from build123d import *

# Parameters (mm, degrees)
SKETCH1_W           = 40
SKETCH1_H           = 40
SKETCH1_R           = 0.9
BOSS_EXTRUDE1_DEPTH = 6
SKETCH11_W          = 40
SKETCH11_H          = 40
SKETCH11_R          = 5
BOSS_EXTRUDE6_DEPTH = 7
SKETCH13_R          = 1.5
SKETCH13_R_2        = 1.395390764
CUT_EXTRUDE5_DEPTH  = 27
SKETCH13_3_R        = 3
SKETCH13_3_R_2      = 1.5
CUT_EXTRUDE6_DEPTH  = 3


with BuildPart() as part:
    # Sketch1 → Boss-Extrude1 (new body)
    with BuildSketch(Plane(origin=(0, 0, 0), x_dir=(0, 1, 0), z_dir=(0, 0, 1))):
        Rectangle(SKETCH1_W, SKETCH1_H)
        with Locations(Location((10.5, 0, 0), (0, 0, 270))):
            Circle(SKETCH1_R, mode=Mode.SUBTRACT)
        with Locations(Location((-10.5, 12.5, 0), (0, 0, 270))):
            Circle(SKETCH1_R, mode=Mode.SUBTRACT)
        with Locations(Location((-10.5, 0, 0), (0, 0, 270))):
            Circle(SKETCH1_R, mode=Mode.SUBTRACT)
        with Locations(Location((10.5, 12.5, 0), (0, 0, 270))):
            Circle(SKETCH1_R, mode=Mode.SUBTRACT)
        Polygon((-5, -13), (-8, -13), (-8, -5), (-5, -5), (-5, 5), (5, 5), (5, -5), (5, -13), align=None, mode=Mode.SUBTRACT)
    extrude(amount=BOSS_EXTRUDE1_DEPTH)

    # Sketch11 → Boss-Extrude6 (add)
    with BuildSketch(Plane.XY.offset(6)):
        Rectangle(SKETCH11_W, SKETCH11_H)
        with Locations(Location((0, 0, 0), (0, 0, 180))):
            Circle(SKETCH11_R, mode=Mode.SUBTRACT)
    extrude(amount=BOSS_EXTRUDE6_DEPTH)

    # Sketch13 → Cut-Extrude5 (cut)
    with BuildSketch(Plane(origin=(0, 0, 0), x_dir=(1, 0, 0), z_dir=(0, 0, -1))):
        with Locations(Location((-6.25, 13.75, 0), (0, 0, 180))):
            Circle(SKETCH13_R)
        with Locations(Location((6.25, 13.75, 0), (0, 0, 180))):
            Circle(SKETCH13_R)
        with Locations(Location((6.25, -13.75, 0), (0, 0, 180))):
            Circle(SKETCH13_R_2)
        with Locations(Location((-6.25, -13.75, 0), (0, 0, 180))):
            Circle(SKETCH13_R)
    extrude(amount=-CUT_EXTRUDE5_DEPTH, mode=Mode.SUBTRACT)

    # Sketch13_3 → Cut-Extrude6 (cut)
    # profile 1 of 4: a face of its own
    with BuildSketch(Plane(origin=(0, 0, 0), x_dir=(1, 0, 0), z_dir=(0, 0, -1))):
        with Locations(Location((-6.25, -13.75, 0), (0, 0, 180))):
            Circle(SKETCH13_3_R)
        with Locations(Location((-6.25, -13.75, 0), (0, 0, 180))):
            Circle(SKETCH13_3_R_2, mode=Mode.SUBTRACT)
    # profile 2 of 4: a face of its own
    with BuildSketch(Plane(origin=(0, 0, 0), x_dir=(1, 0, 0), z_dir=(0, 0, -1))):
        with Locations(Location((6.25, 13.75, 0), (0, 0, 180))):
            Circle(SKETCH13_3_R)
        with Locations(Location((6.25, 13.75, 0), (0, 0, 180))):
            Circle(SKETCH13_3_R_2, mode=Mode.SUBTRACT)
    # profile 3 of 4: a face of its own
    with BuildSketch(Plane(origin=(0, 0, 0), x_dir=(1, 0, 0), z_dir=(0, 0, -1))):
        with Locations(Location((-6.25, 13.75, 0), (0, 0, 180))):
            Circle(SKETCH13_3_R)
        with Locations(Location((-6.25, 13.75, 0), (0, 0, 180))):
            Circle(SKETCH13_3_R_2, mode=Mode.SUBTRACT)
    # profile 4 of 4: a face of its own
    with BuildSketch(Plane(origin=(0, 0, 0), x_dir=(1, 0, 0), z_dir=(0, 0, -1))):
        with Locations(Location((6.25, -13.75, 0), (0, 0, 180))):
            Circle(SKETCH13_3_R)
    extrude(amount=-CUT_EXTRUDE6_DEPTH, mode=Mode.SUBTRACT)


solid = part.part
CAD build for the part. Positions are in the model's coordinates, mm. A direction names the side the tool comes from. Give positions to 0.01 mm unless a question says otherwise; leave off trailing zeros. Loops run counter-clockwise (first coordinate to the right, second up) from the corner with the lowest first, then second, coordinate; pieces in that order, holes last. Notation, with made-up numbers: M -35.75,67 L -24.75,67 A21 ccw -24.75,105 Z; hole C -18,76.25 d5. An arc over 180 degrees is marked long. One line per question, with ' | ' between items. Start each with the question number.
1. Saw through at B-B on y = -13.75. Give the cut face in (x, z), plus the area to 3 significant figures.
2. Saw through at C-C on z = 8. Give the cut face in (x, y).
3. Probe L1, parallel to X at y = 2, z = 3.5; L2, parallel to Y at x = -6.25, z = 9; L3, parallel to Y at x = -6.25, z = 1.2. List the from-to ranges inside material, lowest first. Write a range as from..to.
4. 3-axis set-ups, long thin cutter, end or side, ignore diameter. For faces 5 (the face through (-7.634, -16.412, 1.479)), 6 (the face through (5, 0, 9)): which of +Z, -Z, +X, -X, +Y, -Y reach the whole face in a straight line?
5. Flat gauge pins, fed straight in: pin 1 (1.8 mm diameter, centred on x = 5, y = 14.5, fed in from -Z); pin 2 (1.6 mm diameter, centred on x = 0, y = -10.5, fed in from -Z). Where does each tip first touch, or does it go through?
6. Saw through at D-D on x = 11. Give the cut face in (y, z), plus the area to 3 significant figures.
7. Saw through at A-A on x = 6.25. Give the cut face in (y, z).
8. Two-plate mould, pull along X, no slides. Class faces 1 (the face through (20, 0, 6)), 2 (the face through (5, -7, 3)), 3 (the face through (-9, 0, 0)), 4 (the face through (-0.12, 11.39, 2.96)): pulls with the +X half, pulls with the -X half, needs draft (parallel to the pull), parting line crosses it, or undercut.
Result sheet:
1) outline: M -20,0 L -9.25,0 L -9.25,3 L -7.75,3 L -7.75,13 L -20,13 Z; M -4.75,3 L -3.25,3 L -3.25,0 L 3.25,0 L 3.25,3 L 4.75,3 L 4.75,13 L -4.75,13 Z; M 7.75,3 L 9.25,3 L 9.25,0 L 20,0 L 20,13 L 7.75,13 Z | area: 424 mm^2
2) outline: M -20,-20 L 20,-20 L 20,20 L -20,20 Z; hole C -6.25,-13.75 d3; hole C -6.25,13.75 d3; hole C 0,0 d10; hole C 6.25,-13.75 d3; hole C 6.25,13.75 d2.79
3) L1: x = -20..-5, 13..20 | L2: y = -20..-15.25, -12.25..12.25, 15.25..20 | L3: y = -20..-16.75, -10.75..10.75, 16.75..20
4) face 5: -Z | face 6: +Z, -Z
5) pin 1: stops at z = 3 | pin 2: stops at z = 6
6) outline: M -20,0 L -8,0 L -8,6 L 5,6 L 5,0 L 20,0 L 20,13 L -20,13 Z | area: 442 mm^2
7) outline: M -20,0 L -16.75,0 L -16.75,3 L -15.25,3 L -15.25,13 L -20,13 Z; M -12.25,3 L -10.75,3 L -10.75,0 L -8,0 L -8,6 L 5,6 L 5,0 L 10.75,0 L 10.75,3 L 12.35,3 L 12.35,13 L -12.25,13 Z; M 15.15,3 L 16.75,3 L 16.75,0 L 20,0 L 20,13 L 15.15,13 Z
8) face 1: pulls with the +X half | face 2: undercut | face 3: needs draft | face 4: undercut
